Build history of the part. All positions in model axes, mm. Face numbers are marked on the shaded views. Give positions to 0.01 mm unless a question says otherwise; leave off trailing zeros. Loops run counter-clockwise (first coordinate to the right, second up) from the corner with the lowest first, then second, coordinate; pieces in that order, holes last. Notation, with made-up numbers: (54, -16) -> (69, -16) arc R24 ccw to (69, 4) -> close; hole circle Ø4 at (88.25, 23.5). An arc over 180 degrees is marked (long way). Answer as a JSON object with one key per item and string values. Group by question number.
Q1. Drop flat-ended pins along their axis: pin 1 (4 mm diameter, centred on x = 9.5, z = 19.5, fed in from -Y); pin 2 (2 mm diameter, centred on x = 3, y = 6.5, fed in from +Z); pin 3 (3 mm diameter, centred on y = 3.5, z = 6, fed in from +X). Give the stop position or say it passes through.
Q2. Band-saw the part on B-B, the plane x = 9.75. Write the cut outline in (y, z).
Q3. Wall check: probe 1 along Y at (x, z) = (5.75, 2); probe 2 along Y at (x, z) = (0.25, 9); probe 3 along X at (y, z) = (6.5, 5). Give the ranges that are in metal, low to high. Write a range as from..to.
Q4. Two-plate mould, pull along Y, no slides. Class the marked faces 1 and 2: pulls with the +Y half, pulls with the -Y half, needs draft (parallel to the pull), parting line crosses it, or undercut.
Q5. Band-saw the part on D-D, the plane z = 36.5. Write the cut outline in (x, y), plus the area to 3 significant figures.
Q6. Band-saw the part on A-A, the plane z = 5. Write the cut outline in (x, y).
Q7. Band-saw the part on C-C, the plane y = 5.75. Write the cut outline in (x, z).
from build123d import *

# Parameters (mm, degrees)
BOSS_EXTRUDE1_DEPTH = 20
BOSS_EXTRUDE2_DEPTH = 20
CUT_EXTRUDE1_REACH  = 44.914
SKETCH3_R           = 1.5
SKETCH4_R           = 1.6
CUT_EXTRUDE2_DEPTH  = 43.62188405
CUT_EXTRUDE3_DEPTH  = 43.914158503


with BuildPart() as part:
    # Sketch1 → Boss-Extrude1 (new body)
    with BuildSketch(Plane.XY):
        Polygon((0, 0), (-4.185789452, 7.25), (13.75, 7.25), (13.75, 5.25), (-0.721687836, 5.25), (1.732050808, 1), align=None)
    extrude(amount=BOSS_EXTRUDE1_DEPTH)

    # Sketch2 → Boss-Extrude2 (add)
    with BuildSketch(Plane.XY.offset(20)):
        Polygon((-4.185789452, 7.25), (0, 0), (1.732050808, 1), (-1.876388375, 7.25), align=None)
    extrude(amount=BOSS_EXTRUDE2_DEPTH)

    # Sketch3 → Cut-Extrude1 (cut, up to next)
    with BuildSketch(Plane(origin=(0, 0, 0), x_dir=(0, 0, 1), z_dir=(-0.8660254037844363, -0.5000000000000042, 0)), mode=Mode.PRIVATE) as cut_extrude1_sk1:
        with Locations(Location((2.5, 2.5, 0), (0, 0, 270))):
            Circle(SKETCH3_R)
    cut_extrude1_tool1 = extrude(cut_extrude1_sk1.sketch, amount=-CUT_EXTRUDE1_REACH, mode=Mode.PRIVATE) & part.part
    # Sketch3 → Cut-Extrude1 (cut, up to next)
    with BuildSketch(Plane(origin=(0, 0, 0), x_dir=(0, 0, 1), z_dir=(-0.8660254037844363, -0.5000000000000042, 0)), mode=Mode.PRIVATE) as cut_extrude1_sk2:
        with Locations(Location((37.5, 2.5, 0), (0, 0, 270))):
            Circle(SKETCH3_R)
    cut_extrude1_tool2 = extrude(cut_extrude1_sk2.sketch, amount=-CUT_EXTRUDE1_REACH, mode=Mode.PRIVATE) & part.part
    add(cut_extrude1_tool1.solids().sort_by_distance((-1.25, 2.165064, 2.5))[0], mode=Mode.SUBTRACT)
    add(cut_extrude1_tool2.solids().sort_by_distance((-1.25, 2.165064, 37.5))[0], mode=Mode.SUBTRACT)

    # Sketch4 → Cut-Extrude2 (cut, through all)
    with BuildSketch(Plane.XZ.offset(-5.25)):
        with Locations(Location((9.75, 15, 0), (0, 0, 270))):
            Circle(SKETCH4_R)
        with Locations(Location((9.75, 5, 0), (0, 0, 270))):
            Circle(SKETCH4_R)
    extrude(amount=-CUT_EXTRUDE2_DEPTH, mode=Mode.SUBTRACT)

    # Sketch5 → Cut-Extrude3 (cut, through all)
    with BuildSketch(Plane(origin=(0, 7.25, 0), x_dir=(1, 0, 0), z_dir=(0, 1, 0))):
        Polygon((13.75, -20), (13.75, -10), (12, -20), align=None)
    extrude(amount=-CUT_EXTRUDE3_DEPTH, mode=Mode.SUBTRACT)


solid = part.part
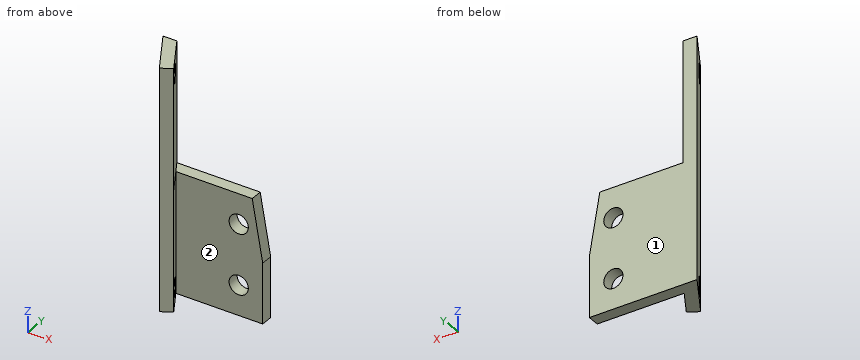
Worked answers:
{
 "1": {"pin 1": "y = 5.25", "pin 2": "z = 20", "pin 3": "x = 1.15"},
 "2": {"outline": "(5.25, 0) -> (7.25, 0) -> (7.25, 3.4) -> (5.25, 3.4) -> close; (5.25, 6.6) -> (7.25, 6.6) -> (7.25, 13.4) -> (5.25, 13.4) -> close; (5.25, 16.6) -> (7.25, 16.6) -> (7.25, 20) -> (5.25, 20) -> close"},
 "3": {"probe 1": "5.25..7.25", "probe 2": "0.14..3.57, 5.25..7.25", "probe 3": "-3.75..8.15, 11.35..13.75"},
 "4": {"face 1": "pulls with the +Y half", "face 2": "undercut"},
 "5": {"outline": "(-4.19, 7.25) -> (-1.81, 3.13) -> (-0.08, 4.13) -> (-1.88, 7.25) -> close; (-0.69, 1.2) -> (0, 0) -> (1.73, 1) -> (1.04, 2.2) -> close", "area": "11.1 mm2"},
 "6": {"outline": "(-4.19, 7.25) -> (0, 0) -> (1.73, 1) -> (-0.72, 5.25) -> (8.15, 5.25) -> (8.15, 7.25) -> close; (11.35, 5.25) -> (13.75, 5.25) -> (13.75, 7.25) -> (11.35, 7.25) -> close"},
 "7": {"outline": "(-3.32, 0) -> (13.75, 0) -> (13.75, 10) -> (12, 20) -> (-1.01, 20) -> (-1.01, 40) -> (-3.32, 40) -> close; hole circle Ø3.2 at (9.75, 5); hole circle Ø3.2 at (9.75, 15)"}
}
